Could you check a few things on this model? Use its own coordinates, in mm. Face numbers are marked on the shaded views. A direction names the side the tool comes from. Give positions to 0.01 mm unless a question says otherwise; leave off trailing zeros. Write each loop counter-clockwise with the first axis right and the second up, starting at its lowest first coordinate (ties: lowest second). Pieces come first, ordered by that corner, then holes. Notation, with made-up numbers: (81, -25.5) - (119, -25.5) arc R21 cw to (119, -9.5) - close; hole circle Ø1 at (66.5, 74). An arc over 180 degrees is marked (long way). Answer in a Markdown table with one row per item.
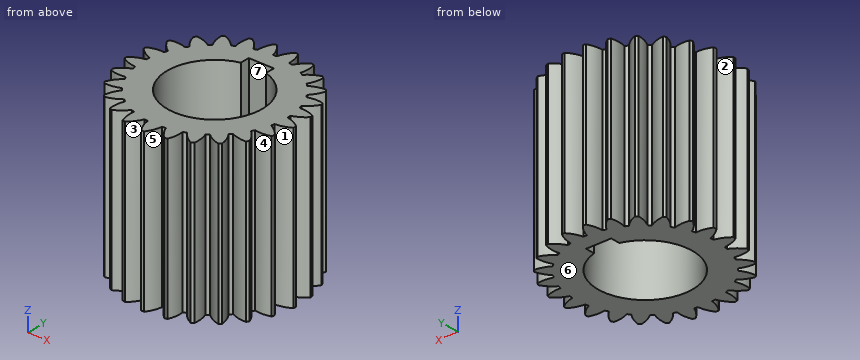
from build123d import *

# Parameters (mm, degrees)
SKETCH1_R           = 27
BOSS_EXTRUDE1_DEPTH = 50
CUT_EXTRUDE1_DEPTH  = 50
CIRPATTERN1_COUNT   = 25
CUT_EXTRUDE2_DEPTH  = 50


with BuildPart() as part:
    # Sketch1 → Boss-Extrude1 (new body)
    with BuildSketch(Plane.XY):
        Circle(SKETCH1_R)
    extrude(amount=BOSS_EXTRUDE1_DEPTH)

    # Sketch3 → Cut-Extrude1 (cut)
    with BuildSketch(Plane.XY.offset(50)):
        with BuildLine():
            Line((3.082235405, 27), (-3.082235405, 27))
            ThreePointArc((-3.082235405, 27), (-1.513981077, 24.920996669), (-0.55457938, 22.5))
            Line((-0.55457938, 22.5), (0.55457938, 22.5))
            ThreePointArc((0.55457938, 22.5), (1.513981077, 24.920996669), (3.082235405, 27))
        make_face()
    cut_extrude1 = extrude(amount=-CUT_EXTRUDE1_DEPTH, mode=Mode.SUBTRACT)

    # CirPattern1: Cut-Extrude1 ×25 about axis
    cirpattern1_axis = Axis((0, 0, 0), (0, 0, 1))
    for i in range(1, CIRPATTERN1_COUNT):
        add(cut_extrude1.rotate(cirpattern1_axis, i * 360 / CIRPATTERN1_COUNT), mode=Mode.SUBTRACT)

    # Sketch4 → Cut-Extrude2 (cut)
    with BuildSketch(Plane.XY.offset(50)):
        with BuildLine():
            Line((-4, 14.456832295), (-4, 17.456832295))
            Line((-4, 17.456832295), (4, 17.456832295))
            Line((4, 17.456832295), (4, 14.456832295))
            ThreePointArc((4, 14.456832295), (0, -15), (-4, 14.456832295))
        make_face()
    extrude(amount=-CUT_EXTRUDE2_DEPTH, mode=Mode.SUBTRACT)


solid = part.part
1) On a 3-axis mill with a long thin cutter (end or side, diameter ignored), from which of +Z, -Z, +X, -X, +Y, -Y can I reach the whole of each face in a straight line? I mean the marked faces 1, 2, 3 and 4. Say none if no direction works.
Check values:
| item | result |
|---|---|
| face 1 | +Z, -Z, +X |
| face 2 | +Z, -Z, -X |
| face 3 | +Z, -Z, -Y |
| face 4 | +Z, -Z |
2) Imagine slicing it at B-B (y = -13). List the corners of the cut face in (x, z) for me.
Check values:
| item | result |
|---|---|
| outline | (-22.54, 0) - (-7.48, 0) - (-7.48, 50) - (-22.54, 50) - close; (7.48, 0) - (22.54, 0) - (22.54, 50) - (7.48, 50) - close |
3) We'd pull the mould along Y, two halves only. Please class the marked faces 5, 6 and 7: +Y half, -Y half, draft (parallel to the pull), parting line (faces both ways), or undercut.
Check values:
| item | result |
|---|---|
| face 5 | -Y half |
| face 6 | draft |
| face 7 | undercut |
4) If I drill on line 1 (Y direction, x = 23.5, z = 13); line 2 (X direction, y = 6.5, z = 16); line 3 (X direction, y = 13, z = 31.5), over which ranges is the centre line in solid material (lowest first)?
Check values:
| item | result |
|---|---|
| line 1 | y = -9.21 to -5.62, -3.51 to 0.62, 2.38 to 6.37, 9.44 to 12.02 |
| line 2 | x = -21.55 to -13.52, 13.52 to 21.55 |
| line 3 | x = -19.13 to -7.48, 7.48 to 19.13 |
5) Imagine slicing it at A-A (y = 0). List the corners of the cut face in (x, z) for me.
Check values:
| item | result |
|---|---|
| outline | (-25.08, 0) - (-15, 0) - (-15, 50) - (-25.08, 50) - close; (15, 0) - (25.08, 0) - (25.08, 50) - (15, 50) - close |
6) Will these pins go through, and if not, where does the flat tip stop? P1, Ø12, axis at x = 9, z = 5.5, coming from the +Y side; P2, Ø0.6, axis at x = 0, z = 32, coming from the +Y side; P3, Ø1.5, axis at y = 16, z = 36, coming from the -X side.
Check values:
| item | result |
|---|---|
| P1 | stops at y = 26.83 |
| P2 | stops at y = 22.5 |
| P3 | stops at x = -21.07 |
